from build123d import *

# Parameters (mm, degrees)
SKETCH1_R                       = 42.5
SKETCH1_R_2                     = 1.6
SKETCH1_R_3                     = 7.5
BOSS_EXTRUDE1_DEPTH             = 3
SKETCH3_R                       = 42.5
SKETCH3_R_2                     = 37.5
SKETCH3_R_3                     = 14.9
SKETCH3_R_4                     = 1.6
SKETCH3_R_5                     = 7.5
BOSS_EXTRUDE2_DEPTH             = 3
BOSS_EXTRUDE3_REACH             = 308.999
SKETCH4_R                       = 1.6
BOSS_EXTRUDE3_DIRECTION_2_REACH = 308.999


with BuildPart() as part:
    # Sketch1 → Boss-Extrude1 (new body)
    with BuildSketch(Plane.XY):
        with Locations((260.117045421, -9.1)):
            Circle(SKETCH1_R)
        with Locations((252.197449472, -1.180404051)):
            Circle(SKETCH1_R_2, mode=Mode.SUBTRACT)
        with Locations((268.036641371, -1.180404051)):
            Circle(SKETCH1_R_2, mode=Mode.SUBTRACT)
        with Locations((252.197449472, -17.019595949)):
            Circle(SKETCH1_R_2, mode=Mode.SUBTRACT)
        with Locations((268.036641371, -17.019595949)):
            Circle(SKETCH1_R_2, mode=Mode.SUBTRACT)
        with Locations((260.117045421, -9.1)):
            Circle(SKETCH1_R_3, mode=Mode.SUBTRACT)
    extrude(amount=BOSS_EXTRUDE1_DEPTH)

    # Sketch3 → Boss-Extrude2 (add)
    # profile 1 of 2: a face of its own
    with BuildSketch(Plane.XY.offset(3)):
        with Locations((260.117045421, -9.1)):
            Circle(SKETCH3_R)
        with Locations((260.117045421, -9.1)):
            Circle(SKETCH3_R_2, mode=Mode.SUBTRACT)
    # profile 2 of 2: a face of its own
    with BuildSketch(Plane.XY.offset(3)):
        with Locations((260.117045421, -9.1)):
            Circle(SKETCH3_R_3)
        with Locations((252.197449472, -17.019595949)):
            Circle(SKETCH3_R_4, mode=Mode.SUBTRACT)
        with Locations((268.036641371, -1.180404051)):
            Circle(SKETCH3_R_4, mode=Mode.SUBTRACT)
        with Locations((268.036641371, -17.019595949)):
            Circle(SKETCH3_R_4, mode=Mode.SUBTRACT)
        with Locations((260.117045421, -9.1)):
            Circle(SKETCH3_R_5, mode=Mode.SUBTRACT)
        with Locations((252.197449472, -1.180404051)):
            Circle(SKETCH3_R_4, mode=Mode.SUBTRACT)
    extrude(amount=BOSS_EXTRUDE2_DEPTH)

    # Boss-Extrude3: up to this face of the body (flat: up to its plane)
    boss_extrude3_end = Plane(part.part.faces().sort_by_distance((218.819126949, -9.1, 6))[0])
    # Sketch4 → Boss-Extrude3 (add, up to the picked face)
    with BuildSketch(Plane.XY.offset(3), mode=Mode.PRIVATE) as boss_extrude3_sk1:
        with BuildLine():
            Line((217.617045421, -9.1), (213.617045421, -9.1))
            ThreePointArc((213.617045421, -9.1), (212.202831859, -9.685786438), (211.617045421, -11.1))
            Line((211.617045421, -11.1), (211.617045421, -13.1))
            ThreePointArc((211.617045421, -13.1), (212.202831859, -14.514213562), (213.617045421, -15.1))
            Line((213.617045421, -15.1), (218.042706448, -15.1))
            ThreePointArc((218.042706448, -15.1), (217.723594239, -12.107539996), (217.617045421, -9.1))
        make_face()
        with Locations((214.67031983, -12.103769998)):
            Circle(SKETCH4_R, mode=Mode.SUBTRACT)
    boss_extrude3_tool1 = split(extrude(boss_extrude3_sk1.sketch, amount=BOSS_EXTRUDE3_REACH, mode=Mode.PRIVATE), bisect_by=boss_extrude3_end, keep=Keep.BOTH, mode=Mode.PRIVATE)
    add(boss_extrude3_tool1.solids().sort_by(Axis((215.617045, -9.187914, 3), (0, 0, 1)))[0])

    # Boss-Extrude3 direction 2: up to this face of the body (flat: up to its plane)
    boss_extrude3_direction_2_end = Plane(part.part.faces().sort_by_distance((218.819126949, -9.1, 0))[0])
    # Sketch4 → Boss-Extrude3 direction 2 (add, up to the picked face)
    with BuildSketch(Plane.XY.offset(3), mode=Mode.PRIVATE) as boss_extrude3_direction_2_sk1:
        with BuildLine():
            Line((217.617045421, -9.1), (213.617045421, -9.1))
            ThreePointArc((213.617045421, -9.1), (212.202831859, -9.685786438), (211.617045421, -11.1))
            Line((211.617045421, -11.1), (211.617045421, -13.1))
            ThreePointArc((211.617045421, -13.1), (212.202831859, -14.514213562), (213.617045421, -15.1))
            Line((213.617045421, -15.1), (218.042706448, -15.1))
            ThreePointArc((218.042706448, -15.1), (217.723594239, -12.107539996), (217.617045421, -9.1))
        make_face()
        with Locations((214.67031983, -12.103769998)):
            Circle(SKETCH4_R, mode=Mode.SUBTRACT)
    boss_extrude3_direction_2_tool1 = split(extrude(boss_extrude3_direction_2_sk1.sketch, amount=-BOSS_EXTRUDE3_DIRECTION_2_REACH, mode=Mode.PRIVATE), bisect_by=boss_extrude3_direction_2_end, keep=Keep.BOTH, mode=Mode.PRIVATE)
    add(boss_extrude3_direction_2_tool1.solids().sort_by(Axis((215.617045, -9.187914, 3), (0, 0, -1)))[0])


solid = part.part
Verification items for the finished model (mm, model axes). A direction names the side the tool comes from. Give positions to 0.01 mm unless a question says otherwise; leave off trailing zeros. Write each loop counter-clockwise with the first axis right and the second up, starting at its lowest first coordinate (ties: lowest second). Pieces come first, ordered by that corner, then holes. Notation, with made-up numbers: M 22.5,56.5 L 39.5,56.5 A31 ccw 39.5,83.5 Z; hole C 44.5,54.25 d11. An arc over 180 degrees is marked long. Put each result on its own line as item: value. Start each with the question number.
1. Go/stop test with flat-tipped pins: pin 1 Ø2 at (x, z) = (282, 3.5) entering from +Y; pin 2 Ø2 at (x, z) = (216.5, 3) entering from -Y; pin 3 Ø2 at (x, z) = (262.5, 4) entering from +Y. Record where each tip stops, or that it passes through.
2. Scan lines: line 1 along X through (y, z) = (-9, 1.5); line 2 along X through (y, z) = (25, 3.1); line 3 along Y through (x, z) = (261, 4.2). Record each from-to range of solid material in increasing order. Write a range as [from, to].
3. Section check D-D (y = -21.5). Record the cut outline in (x, z).
4. Section check C-C (x = 237.5). Record the cut outline in (y, z).
5. Draft check along Y on faces 1 (the face through (216, -15.1, 3)), 2 (the face through (250.6, -1.1, 3)), 3 (the face through (260, 29, 6)). Enter one of: +Y half, -Y half, draft (parallel to the pull), parting line (faces both ways), or undercut.
6. Section check B-B (y = 26.5). Record the cut outline in (x, z), and give its area (3 significant figures).
7. Set-up check for faces 4 (the face through (266.44, -16.95, 2.96)), 5 (the face through (216, -9.1, 3)), 6 (the face through (276, -9, 3)): record each of +Z, -Z, +X, -X, +Y, -Y from which the full face is reachable in a straight line by a thin tool's end or side.
8. Section check A-A (z = 3.95). Give the number of separate pieces and of enclosed holes in the cut face, and give its area (3 significant figures).
Answer list:
1. pin 1: y = 27.92
1. pin 2: y = -15.1
1. pin 3: y = 33.38
2. line 1: [217.62, 252.62], [267.62, 302.62]
2. line 2: [234.75, 244.51], [275.72, 285.48]
2. line 3: [-51.59, -46.59], [-23.97, -16.55], [-1.65, 5.77], [28.39, 33.39]
3. outline: M 219.47,0 L 300.77,0 L 300.77,6 L 295.51,6 L 295.51,3 L 268.38,3 L 268.38,6 L 251.86,6 L 251.86,3 L 224.73,3 L 224.73,6 L 219.47,6 Z
4. outline: M -45.08,0 L 26.88,0 L 26.88,6 L 20.81,6 L 20.81,3 L -39.01,3 L -39.01,6 L -45.08,6 Z
5. face 1: -Y half
5. face 2: undercut
5. face 3: draft
6. outline: M 236.9,0 L 283.33,0 L 283.33,6 L 271.9,6 L 271.9,3 L 248.33,3 L 248.33,6 L 236.9,6 Z
6. area: 208 mm2
7. face 4: +Z, -Z
7. face 5: +Z, -Z, -X, +Y
7. face 6: +Z
8. separate pieces: 2
8. enclosed holes: 7
8. area: 1,770 mm2
